Job drawing, mm, ordinate dimensions from the low corner. One solid piece. Coordinates: 2 decimals unless noted, no trailing zeros. Loops run counter-clockwise (first coordinate to the right, second up) from the corner with the lowest first, then second, coordinate; pieces in that order, holes last. Notation, with made-up numbers: M -25,73.25 L 27,73.25 A15 ccw 27,87.25 Z; hole C 51,43 d7. An arc over 180 degrees is marked long. Write each question's results on one line, items separated by ' | '. Start each with the question number.
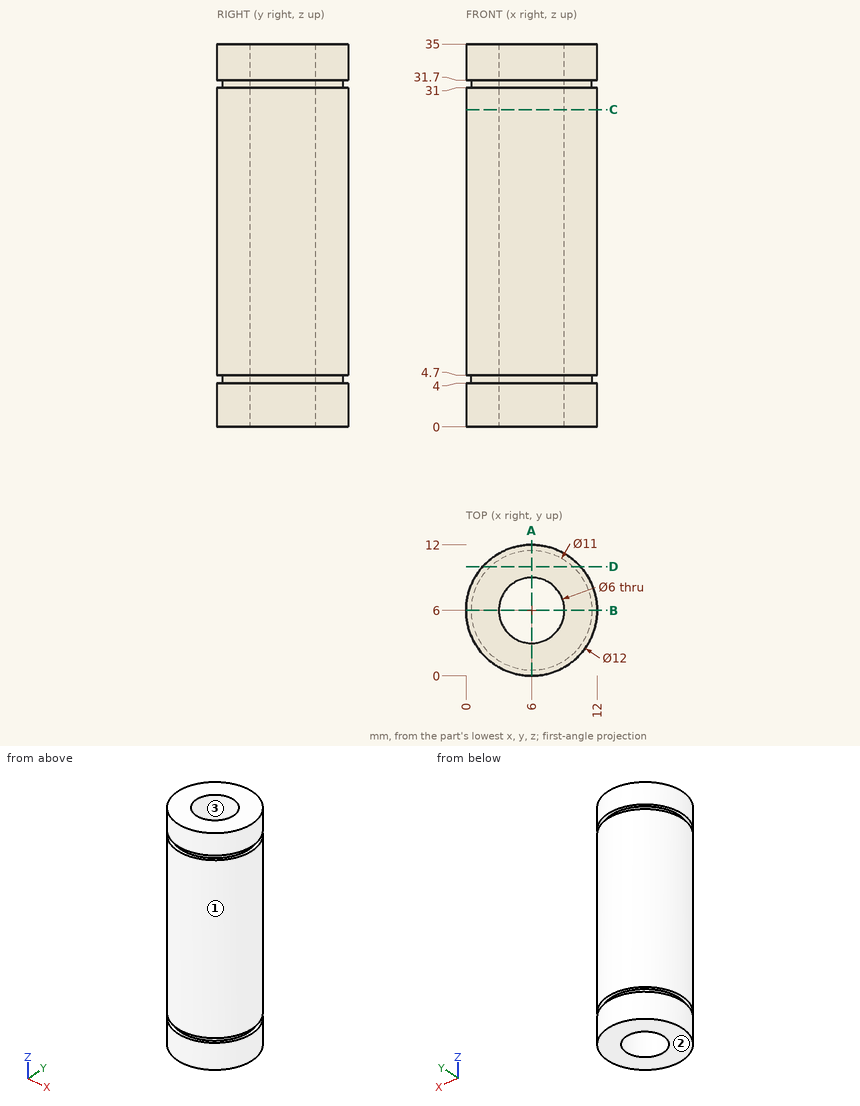
1. Mould opens along X. For the marked faces 1, 2 and 3 say: +X half, -X half, draft (parallel to the pull), parting line (faces both ways), or undercut.
2. Band-saw the part on D-D, the plane y = 10. List the corners of the cut face in (x, z), plus the area to 3 significant figures.
3. Pin check, flat tips, straight feed: pin 1 (3 mm diameter, centred on y = 2.5, z = 19.5, fed in from -X); pin 2 (1 mm diameter, centred on x = 3, z = 18, fed in from -Y); pin 3 (1.5 mm diameter, centred on y = 3, z = 22.5, fed in from -X). Stop position of each tip, or through.
4. Wall check: line 1 along Y through (x, z) = (6, 7.5); line 2 along Y through (x, z) = (4, 25.5); line 3 along X through (y, z) = (10.75, 8). Give the ranges that are in metal, low to high.
5. Band-saw the part on C-C, the plane z = 29. List the corners of the cut face in (x, y).
6. Band-saw the part on A-A, the plane x = 6. List the corners of the cut face in (y, z), plus the area to 3 significant figures.
Checked values:
1) face 1: parting line | face 2: draft | face 3: undercut
2) outline: M 1.53,0 L 10.47,0 L 10.47,4 L 9.77,4 L 9.77,4.7 L 10.47,4.7 L 10.47,31 L 9.77,31 L 9.77,31.7 L 10.47,31.7 L 10.47,35 L 1.53,35 L 1.53,31.7 L 2.23,31.7 L 2.23,31 L 1.53,31 L 1.53,4.7 L 2.23,4.7 L 2.23,4 L 1.53,4 Z | area: 311 mm²
3) pin 1: x = 0.34 | pin 2: y = 0.55 | pin 3: x = 0.44
4) line 1: 0 to 3, 9 to 12 | line 2: 0.34 to 3.76, 8.24 to 11.66 | line 3: 2.33 to 9.67
5) outline: C 6,6 d12; hole C 6,6 d6
6) outline: M 0,0 L 3,0 L 3,35 L 0,35 L 0,31.7 L 0.5,31.7 L 0.5,31 L 0,31 L 0,4.7 L 0.5,4.7 L 0.5,4 L 0,4 Z; M 9,0 L 12,0 L 12,4 L 11.5,4 L 11.5,4.7 L 12,4.7 L 12,31 L 11.5,31 L 11.5,31.7 L 12,31.7 L 12,35 L 9,35 Z | area: 209 mm²
